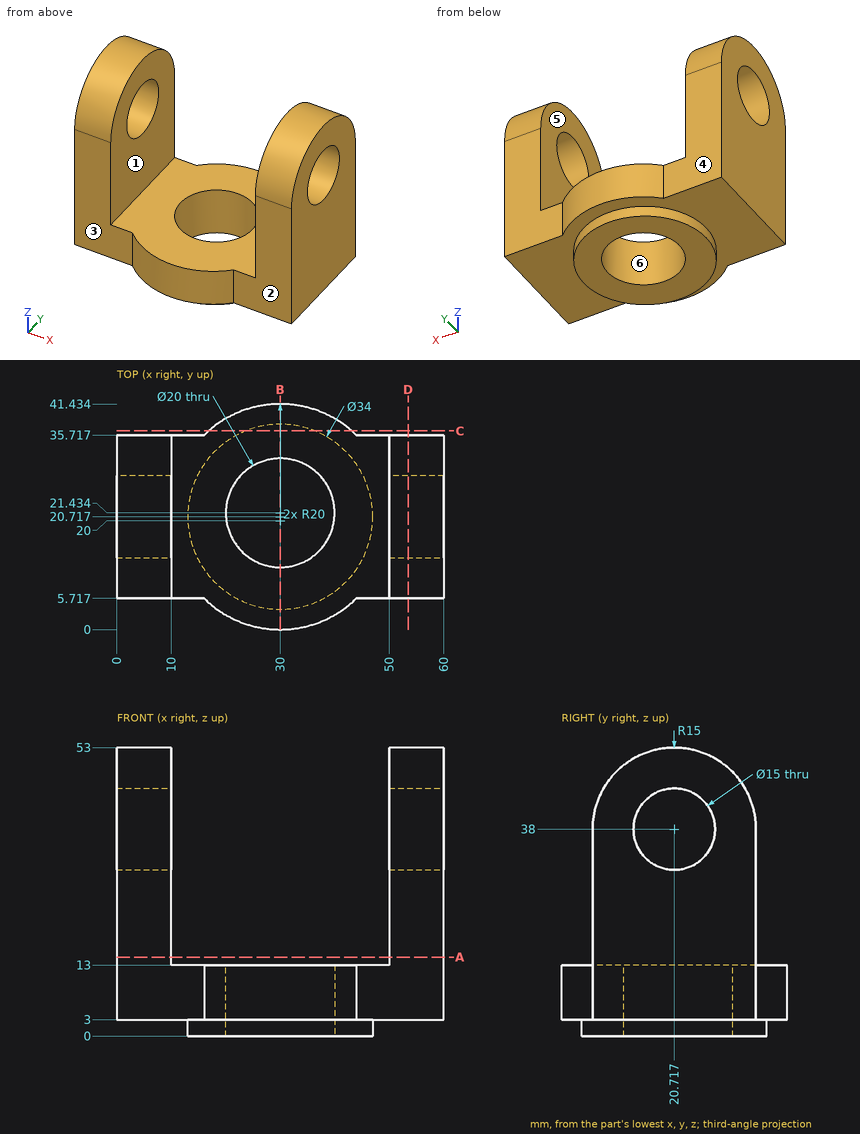
Design review of the part shown in the three views and the two pictorial views. Dimensions are in mm from the part's minimum x, y and z. A direction names the side the tool comes from. Give positions to 0.01 mm unless a question says otherwise; leave off trailing zeros. Write each loop counter-clockwise with the first axis right and the second up, starting at its lowest first coordinate (ties: lowest second). Pieces come first, ordered by that corner, then holes. Notation, with made-up numbers: M -30.5,33.5 L 25.5,33.5 A20 cw 25.5,69.5 Z; hole C 19,46 d4. An arc over 180 degrees is marked long. Answer in a Markdown table with one row per item.
Item 1: Draft analysis for pull direction Y (two halves, no side actions). For the marked faces 4, 5 and 6, state which applies: +Y half, -Y half, draft (parallel to the pull), parting line (faces both ways), or undercut.
Check sheet entries:
| item | result |
|---|---|
| face 4 | +Y half |
| face 5 | draft |
| face 6 | undercut |
Item 2: Add section D-D on x = 53.5. Give the boundary of the cut face in (y, z), plus the area to 3 significant figures.
Check sheet entries:
| item | result |
|---|---|
| outline | M 5.72,3 L 35.72,3 L 35.72,38 A15 ccw 5.72,38 Z; hole C 20.72,38 d15 |
| area | 1,230 mm2 |
Item 3: Add section C-C on y = 36.5. Give the boundary of the cut face in (x, z), plus the area to 3 significant figures.
Check sheet entries:
| item | result |
|---|---|
| outline | M 16.85,3 L 23.68,3 L 23.68,0 L 36.32,0 L 36.32,3 L 43.15,3 L 43.15,13 L 16.85,13 Z |
| area | 301 mm2 |
Item 4: For P1, Ø2, axis at x = 54, z = 33.5, coming from the -Y side; P2, Ø4, axis at x = 45, y = 15, coming from the +Z side; P3, Ø13, axis at x = 48.5, z = 13.5, coming from the +Y side, all flat-tipped, find the tip position at first contact; note any pin that passes through.
Check sheet entries:
| item | result |
|---|---|
| P1 | y = 5.72 |
| P2 | z = 13 |
| P3 | y = 37.42 |
Item 5: Tool access review of the marked faces 1, 2 and 3: name each direction out of +Z, -Z, +X, -X, +Y, -Y from which nothing blocks a thin tool from reaching the whole face with its end or side.
Check sheet entries:
| item | result |
|---|---|
| face 1 | +Z, +Y, -Y |
| face 2 | +Z, -Z, +X, -Y |
| face 3 | +Z, -Z, -X, -Y |
Item 6: Add section A-A on z = 14.5. Give the boundary of the cut face in (x, y), plus the area to 3 significant figures.
Check sheet entries:
| item | result |
|---|---|
| outline | M 0,5.72 L 10,5.72 L 10,35.72 L 0,35.72 Z; M 50,5.72 L 60,5.72 L 60,35.72 L 50,35.72 Z |
| area | 600 mm2 |
Item 7: For line 1 along X through (y, z) = (29, 27.5); line 2 along Y through (x, z) = (6, 38); line 3 along Z through (x, y) = (30.5, 5.5), list the stretches that pass through material, from the lowest coordinate up.
Check sheet entries:
| item | result |
|---|---|
| line 1 | 0 to 10, 50 to 60 |
| line 2 | 5.72 to 13.22, 28.22 to 35.72 |
| line 3 | 0 to 13 |
Item 8: Add section B-B on x = 30. Give the boundary of the cut face in (y, z).
Check sheet entries:
| item | result |
|---|---|
| outline | M 0,3 L 3.72,3 L 3.72,0 L 11.43,0 L 11.43,13 L 0,13 Z; M 31.43,0 L 37.72,0 L 37.72,3 L 41.43,3 L 41.43,13 L 31.43,13 Z |
